The listing builds one solid part. Answer for the finished solid, in the listing's coordinates (mm). A direction names the side the tool comes from. Give positions to 0.01 mm unless a question says otherwise; leave off trailing zeros. Write each loop counter-clockwise with the first axis right and the second up, starting at its lowest first coordinate (ties: lowest second). Pieces come first, ordered by that corner, then holes. Notation, with made-up numbers: (54.5, 25.5) -> (69.5, 25.5) arc R32 cw to (69.5, 60.5) -> close; hole circle Ø8 at (41, 86.25). An arc over 180 degrees is marked (long way). Use CSV: the item, a comma, the result in double quotes. Start each with the question number.
from build123d import *

# Parameters (mm, degrees)
F1_DEPTH = 68.326
F2_W     = 29.21
F2_H     = 14.351
F2_W_2   = 20.066
F2_H_2   = 51.054
F3_DEPTH = 140.2725
F9_DEPTH = 19.05


with BuildPart() as f1:
    # F0 (on Front) → F1 (new body)
    with BuildSketch(Plane.XZ):
        with BuildLine():
            Line((-140.2715, 0), (0, 0))
            Line((0, 0), (0, 28.575))
            Line((0, 28.575), (-104.1369961518, 77.1348788028))
            ThreePointArc((-104.1369961518, 77.1348788028), (-128.518910052, 75.5368037358), (-140.2715, 54.1146610121))
            Line((-140.2715, 54.1146610121), (-140.2715, 0))
        make_face()
    extrude(amount=F1_DEPTH)

    # F2 (on face) → F3 (cut, through all)
    with BuildSketch(Plane.YZ):
        with Locations((-53.721, 7.1755)):
            Rectangle(F2_W, F2_H)
        with Locations((-58.293, 54.102)):
            Rectangle(F2_W_2, F2_H_2)
    extrude(amount=-F3_DEPTH, mode=Mode.SUBTRACT)

    # F5 (on offset) → F6 (revolve, cut)
    with BuildSketch(Plane.XZ.offset(22.225)):
        Polygon((-71.1155433788, 30.3478274527), (-62.0181519767, 19.5059785661), (-47.4676890845, 50.709546935), (-59.0928990688, 56.1304713784), align=None)
    revolve(axis=Axis((-54.7429205306, -22.225, 35.1077627505), (0.4226182617, 0, 0.906307787)), mode=Mode.SUBTRACT)

    # F8 (on offset) → F9 (cut)
    with BuildSketch(Plane.XZ.offset(15.748)):
        Polygon((-140.2715, 82.0435324035), (-140.2715, 38.0492), (-83.1215, 38.0492), (-71.9043142808, 62.1045324035), (-71.9043142808, 82.0435324035), align=None)
    extrude(amount=F9_DEPTH, mode=Mode.SUBTRACT)


solid = f1.part
Q1. The mould has two halves that part along Y. Classify faces 5 (the face through (-85, -48.26, 48)), 6 (the face through (-71, -19, 0)), 7 (the face through (-44.99, -30.89, 33.64)), 8 (the face through (-87, 0, 31)): +Y half, -Y half, draft (parallel to the pull), parting line (faces both ways), or undercut.
Q2. Section B-B on z = 5.5 is taken. Give the vertices of the cut face in (x, y), then the cut area to 3 significant figures.
Q3. Section A-A on z = 69 is taken. Give the vertices of the cut face in (x, y).
Q4. Straight lines are drawn through the part: L1, parallel to Y at x = -126.5, z = 61.5; L2, parallel to Y at x = -12, z = 12; L3, parallel to Z at x = -28, y = -63.5 (3 decimals). For each, find the intervals that lie inside material, in ascending order.
Q5. Section D-D on x = -102.5 is taken. Give the vertices of the cut face in (y, z) (3 decimals).
Q6. Section C-C on y = -5 is taken. Give the vertices of the cut face in (x, z) (1 decimal), then the cut area to 3 significant figures.
Q7. Flat-ended cylindrical pins translate along their axes: pin 1 Ø11.5 at (x, z) = (-72, 8.5) entering from -Y; pin 2 Ø5 at (x, y) = (-96, -46) entering from -Z; pin 3 Ø21 at (x, y) = (-116.5, -23.5) entering from +Z. Find the tip coordinate at first contact, or state that the pin passes through.
Q8. For faces 1 (the face through (-62.417, -21.986, 20.012)), 2 (the face through (-69, -58, 28.575)), 3 (the face through (-69, -39.116, 7)), 4 (the face through (-107, -15.748, 54)), determine the directions among +Z, -Z, +X, -X, +Y, -Y from which every point of the face is accessible in a straight line to the end or side of a thin tool.
Output:
1,face 5,"-Y half"
1,face 6,"draft"
1,face 7,"undercut"
1,face 8,"+Y half"
2,outline,"(-140.27, -39.12) -> (0, -39.12) -> (0, 0) -> (-140.27, 0) -> close"
2,area,"5,490 mm²"
3,outline,"(-135.45, -48.26) -> (-86.69, -48.26) -> (-86.69, -34.8) -> (-135.45, -34.8) -> close; (-135.45, -15.75) -> (-86.69, -15.75) -> (-86.69, 0) -> (-135.45, 0) -> close"
4,L1,"-48.26 to -34.8, -15.75 to 0"
4,L2,"-39.12 to 0"
4,L3,"14.351 to 28.575"
5,outline,"(-68.326, 14.351) -> (-39.116, 14.351) -> (-39.116, 0) -> (0, 0) -> (0, 76.372) -> (-15.748, 76.372) -> (-15.748, 38.049) -> (-34.798, 38.049) -> (-34.798, 76.372) -> (-48.26, 76.372) -> (-48.26, 28.575) -> (-68.326, 28.575) -> close"
6,outline,"(-140.3, 0) -> (0, 0) -> (0, 28.6) -> (-104.1, 77.1) arc R25.4 ccw to (-140.3, 54.1) -> close"
6,area,"8,230 mm²"
7,pin 1,"y = -39.12"
7,pin 2,"z = 14.35"
7,pin 3,"z = 79.51"
8,face 1,"none"
8,face 2,"+Z, +X, -X, -Y"
8,face 3,"-Z, +X, -X, -Y"
8,face 4,"+Z, -X"
